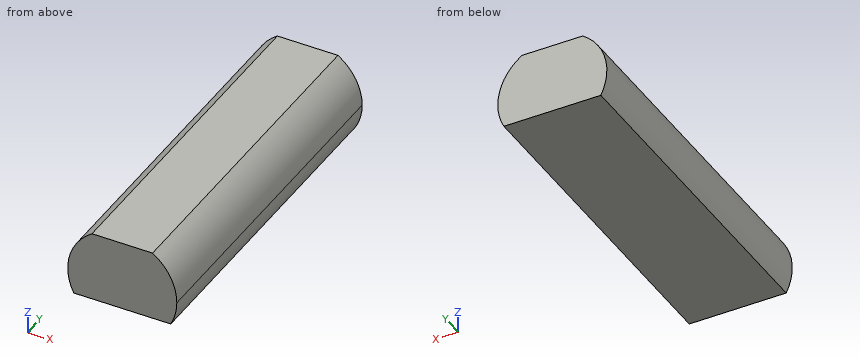
from build123d import *

# Parameters (mm, degrees)
F1_DEPTH = 83.82


with BuildPart() as f1:
    # F0 (on Front) → F1 (new body)
    with BuildSketch(Plane.XZ):
        with BuildLine():
            ThreePointArc((12, -6.698898), (13.119642, -3.696221), (13.5, -0.51424))
            ThreePointArc((13.5, -0.51424), (11.905881, 5.849721), (7.5, 10.710732))
            Line((7.5, 10.710732), (-7.5, 10.710732))
            ThreePointArc((-7.5, 10.710732), (-13.070436, 2.864175), (-12, -6.698898))
            Line((-12, -6.698898), (12, -6.698898))
        make_face()
    extrude(amount=F1_DEPTH)


solid = f1.part
Could you check a few things on this model? Use its own coordinates, in mm. Round coordinates to 2 decimals unless told otherwise and drop trailing zeros. Write each loop counter-clockwise with the first axis right and the second up, starting at its lowest first coordinate (ties: lowest second). Pieces come first, ordered by that corner, then holes. Notation, with made-up numbers: (-39, -19) -> (10, -19) arc R22 ccw to (10, 3) -> close; hole circle Ø9 at (56, 57.5). An arc over 180 degrees is marked (long way). Use a Markdown table: item, result.
1. If we section it at B-B (z = 3.75): List the corners of the cut face in (x, y) for me.
Answer key:
| item | result |
|---|---|
| outline | (-12.81, -83.82) -> (12.81, -83.82) -> (12.81, 0) -> (-12.81, 0) -> close |
2. Please list where these lines run through material, in increasing order: probe 1 along Z at (x, y) = (10.5, -36.5); probe 2 along Z at (x, y) = (-10, -43); probe 3 along X at (y, z) = (-36.5, 2.5).
Answer key:
| item | result |
|---|---|
| probe 1 | z = -6.7 to 7.97 |
| probe 2 | z = -6.7 to 8.55 |
| probe 3 | x = -13.16 to 13.16 |
3. If we section it at A-A (y = -25): List the corners of the cut face in (x, z) for me, then the cut area to 3 significant figures.
Answer key:
| item | result |
|---|---|
| outline | (-12, -6.7) -> (12, -6.7) arc R13.5 ccw to (13.5, -0.51) arc R13.5 ccw to (7.5, 10.71) -> (-7.5, 10.71) arc R13.5 ccw to start |
| area | 424 mm^2 |
4. If we section it at C-C (x = -10): List the corners of the cut face in (y, z) for me, then the cut area to 3 significant figures.
Answer key:
| item | result |
|---|---|
| outline | (-83.82, -6.7) -> (0, -6.7) -> (0, 8.55) -> (-83.82, 8.55) -> close |
| area | 1,280 mm^2 |
